Design review of the part shown in the three views and the two pictorial views. Dimensions are in mm from the part's minimum x, y and z. Round coordinates to 2 decimals unless told otherwise and drop trailing zeros. Order: outer loops, then holes, each group sorted by start corner. A loop starts at its lowest first (then second) coordinate and runs counter-clockwise, first axis right, second up.
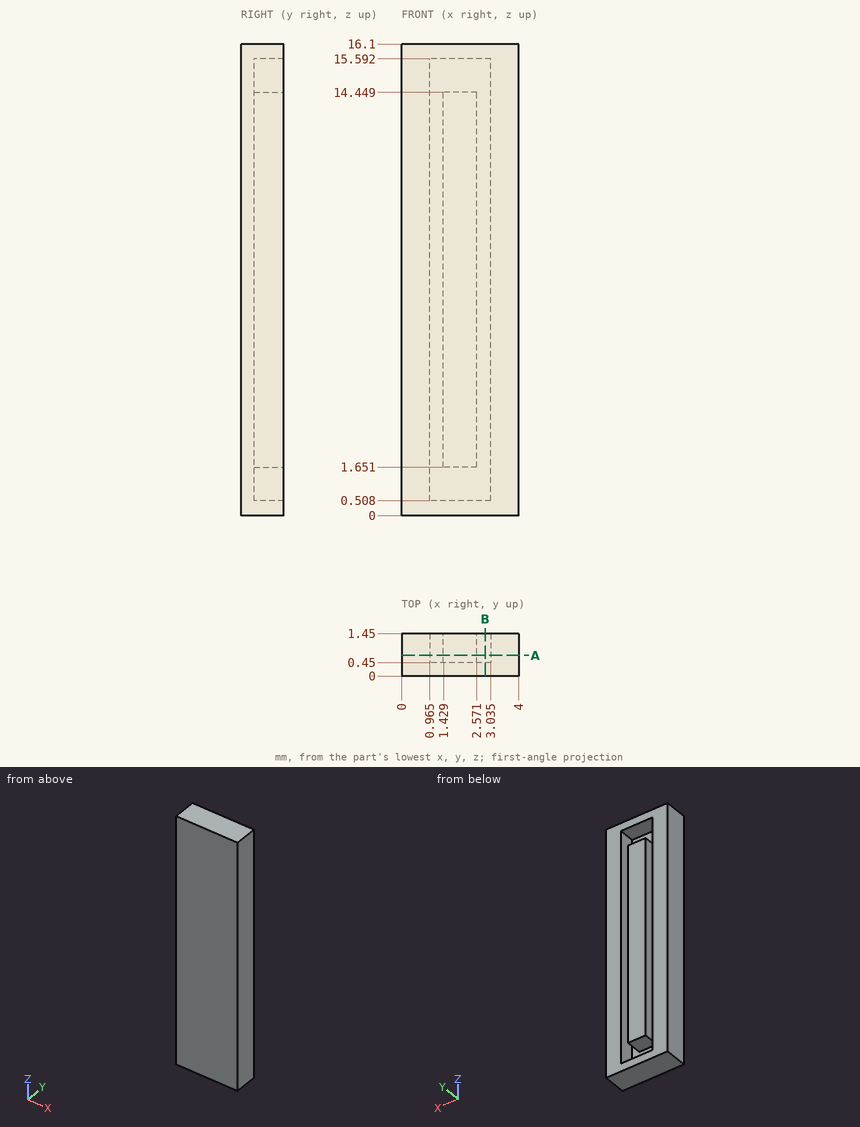
(1) Wall thickness on L1, parallel to X at y = 1, z = 6.25 (1 decimal); L2, parallel to Z at x = 2.2, y = 0.6; L3, parallel to X at y = 1, z = 1.5 (1 decimal): over which ranges is each line inside the solid? List them lowest first.
(2) Add section A-A on y = 0.7. Count the separate pieces of the cut face and the enclosed holes in it.
(3) Add section B-B on x = 2.85. Give the boundary of the cut face in (y, z).
Here are the results:
1. L1: x = 0 to 1, 1.4 to 2.6, 3 to 4
1. L2: z = 0 to 0.51, 1.65 to 14.45, 15.59 to 16.1
1. L3: x = 0 to 1, 3 to 4
2. separate pieces: 2
2. enclosed holes: 1
3. outline: (0, 0) - (1.45, 0) - (1.45, 0.51) - (0.45, 0.51) - (0.45, 15.59) - (1.45, 15.59) - (1.45, 16.1) - (0, 16.1) - close
